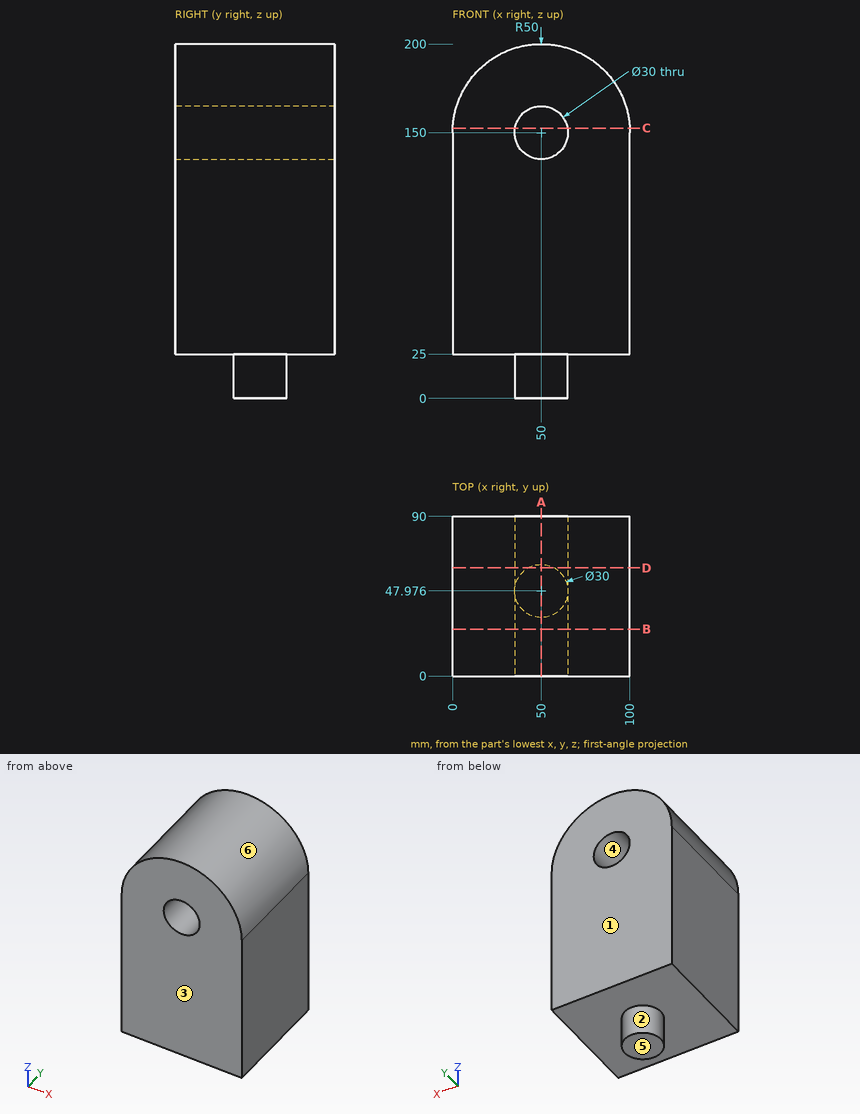
Job drawing, mm, ordinate dimensions from the low corner. One solid piece. A direction names the side the tool comes from. Coordinates: 2 decimals unless noted, no trailing zeros. Loops run counter-clockwise (first coordinate to the right, second up) from the corner with the lowest first, then second, coordinate; pieces in that order, holes last. Notation, with made-up numbers: (50, 50) - (87, 50) arc R9 cw to (87, 54) - close; hole circle Ø7 at (71.25, 22.25). An arc over 180 degrees is marked (long way). Answer as a JSON object with one key per item and string values. Group by question number.
(1) Flat gauge pins, fed straight in: pin 1 (5 mm diameter, centred on y = 17.5, z = 103.5, fed in from -X); pin 2 (5 mm diameter, centred on x = 39.5, y = 66.5, fed in from -Z); pin 3 (1.5 mm diameter, centred on x = 82, y = 16, fed in from +Z). Where does each tip first touch, or does it go through?
(2) Two-plate mould, pull along Z, no slides. Class the marked faces 3, 4, 5 and 6: released by +Z, released by -Z, zero draft, split by the parting line, or undercut.
(3) Tool access for the marked faces 1 and 2: list every direction of +Z, -Z, +X, -X, +Y, -Y with a clear straight run to the whole face (end or side of a thin tool).
(4) Cut at B-B (y = 26.5). Give the cut face in (x, z).
(5) Cut at C-C (z = 152.5). Give the cut face in (x, y), then the cut area to 3 significant figures.
(6) Probe line 1 along Z through (x, y) = (50, 27.5); line 2 along X through (y, z) = (39.5, 150); line 3 along Z through (x, y) = (50, 55.5). List the from-to ranges inside material, lowest first.
(7) Cut at A-A (x = 50). Give the cut face in (y, z), then the cut area to 3 significant figures.
(8) Cut at D-D (y = 61). Give the cut face in (x, z), then the cut area to 3 significant figures.
Geometry says:
{
 "1": {"pin 1": "stops at x = 0", "pin 2": "stops at z = 25", "pin 3": "stops at z = 189.03"},
 "2": {"face 3": "zero draft", "face 4": "undercut", "face 5": "released by -Z", "face 6": "released by +Z"},
 "3": {"face 1": "+Z, -Z, +X, -X, +Y", "face 2": "-Z"},
 "4": {"outline": "(0, 25) - (100, 25) - (100, 150) arc R50 ccw to (0, 150) - close; hole circle Ø30 at (50, 150)"},
 "5": {"outline": "(0.06, 0) - (35.21, 0) - (35.21, 90) - (0.06, 90) - close; (64.79, 0) - (99.94, 0) - (99.94, 90) - (64.79, 90) - close", "area": "6,330 mm^2"},
 "6": {"line 1": "z = 25 to 135, 165 to 200", "line 2": "x = 0 to 35, 65 to 100", "line 3": "z = 0 to 135, 165 to 200"},
 "7": {"outline": "(0, 25) - (32.98, 25) - (32.98, 0) - (62.98, 0) - (62.98, 25) - (90, 25) - (90, 135) - (0, 135) - close; (0, 165) - (90, 165) - (90, 200) - (0, 200) - close", "area": "13,800 mm^2"},
 "8": {"outline": "(0, 25) - (42.56, 25) - (42.56, 0) - (57.44, 0) - (57.44, 25) - (100, 25) - (100, 150) arc R50 ccw to (0, 150) - close; hole circle Ø30 at (50, 150)", "area": "16,100 mm^2"}
}
